Check sheet for the modelled part. Datum: model origin and axes. Units: mm. A direction names the side the tool comes from. Give positions to 0.01 mm unless a question says otherwise; leave off trailing zeros. Order: outer loops, then holes, each group sorted by start corner. A loop starts at its lowest first (then second) coordinate and runs counter-clockwise, first axis right, second up.
```python
from build123d import *

# Parameters (mm, degrees)
F0_R     = 1.5
F1_DEPTH = 2.5
F2_R     = 1


with BuildPart() as f1:
    # F0 (on Front) → F1 (new body)
    with BuildSketch(Plane.XZ):
        with BuildLine():
            ThreePointArc((5, 36.559677), (-0.000826, -36.9), (-4.998364, 36.559901))
            Line((-4.998364, 36.559901), (-5, 36.9))
            Line((-5, 36.9), (-5, 42.204858))
            Line((-5, 42.204858), (-5, 46.9))
            Line((-5, 46.9), (-7.5, 46.9))
            Line((-7.5, 46.9), (-10, 46.9))
            Line((-10, 46.9), (-10, 41.306779))
            ThreePointArc((-10, 41.306779), (0, -42.5), (10, 41.306779))
            Line((10, 41.306779), (10, 46.9))
            Line((10, 46.9), (7.5, 46.9))
            Line((7.5, 46.9), (5, 46.9))
            Line((5, 46.9), (5, 42.204858))
            Line((5, 42.204858), (5, 36.9))
            Line((5, 36.9), (5, 36.559677))
        make_face()
        with Locations((-7.5, 44.552429)):
            Circle(F0_R, mode=Mode.SUBTRACT)
        with Locations((7.5, 44.552429)):
            Circle(F0_R, mode=Mode.SUBTRACT)
    extrude(amount=F1_DEPTH)

    # F2
    f2_edges = [f1.edges().sort_by_distance(p)[0] for p in [
        (-10, -1.25, 46.9),
        (-5, -1.25, 46.9),
        (5, -1.25, 46.9),
        (10, -1.25, 46.9),
        (5, -1.25, 36.559677),
        (-4.998364, -1.25, 36.559901),
    ]]
    fillet(f2_edges, radius=F2_R)


solid = f1.part
```
Q1. Sectioned sample at A-A, the plane z = 0. Record the cut outline in (x, y).
Q2. Sectioned sample at C-C, the plane x = 22. Record the cut outline in (y, z).
Q3. Material ranges on line 1 (Z direction, x = -7.5, y = -0.9); line 2 (X direction, y = -2, z = 0); line 3 (Z direction, x = -28, y = -0.45), recorded low to high.
Q4. Tool access check on faces 4 (the flat face through (-5, -1, 42)), 5 (the flat face through (-10, -1, 44)), 6 (the flat face through (8, -1, 46.9)). Record the directions out of +Z, -Z, +X, -X, +Y, -Y that give a thin tool (end or side, any length) a straight path to the whole face; none if there is none.
Q5. Go/stop test with flat-tipped pins: P1, Ø1.2, axis at y = -1, z = 43, coming from the -X side; P2, Ø0.8, axis at y = -0.5, z = 44, coming from the +X side; P3, Ø0.8, axis at y = -1.5, z = 39.5, coming from the -X side. Record where each tip stops, or that it passes through.
Q6. Sectioned sample at B-B, the plane x = 7.5. Record the cut outline in (y, z).
Q7. Sectioned sample at D-D, the plane y = -1.95. Count the separate pieces of the cut face and the enclosed holes in it, plus the area to 3 significant figures.
Q8. Draft check along X on faces 1 (the flat face through (10, -1, 44)), 2 (the cylindrical face through (-1.727, -1.232, -42.465)), 3 (the flat face through (5, -1, 42)). Enter one of: pulls with the +X half, pulls with the -X half, needs draft (parallel to the pull), parting line crosses it, or undercut.
Filled in:
1. outline: (-42.5, -2.5) - (-36.9, -2.5) - (-36.9, 0) - (-42.5, 0) - close; (36.9, -2.5) - (42.5, -2.5) - (42.5, 0) - (36.9, 0) - close
2. outline: (-2.5, -36.36) - (0, -36.36) - (0, -29.62) - (-2.5, -29.62) - close; (-2.5, 29.62) - (0, 29.62) - (0, 36.36) - (-2.5, 36.36) - close
3. line 1: z = -41.83 to -36.13, 36.13 to 43.05, 46.05 to 46.9
3. line 2: x = -42.5 to -36.9, 36.9 to 42.5
3. line 3: z = -31.97 to -24.03, 24.03 to 31.97
4. face 4: +Z, +Y, -Y
4. face 5: +Z, -X, +Y, -Y
4. face 6: +Z, +X, -X, +Y, -Y
5. P1: stops at x = -10
5. P2: stops at x = 10
5. P3: stops at x = -16.66
6. outline: (-2.5, -41.83) - (0, -41.83) - (0, -36.13) - (-2.5, -36.13) - close; (-2.5, 36.13) - (0, 36.13) - (0, 43.05) - (-2.5, 43.05) - close; (-2.5, 46.05) - (0, 46.05) - (0, 46.9) - (-2.5, 46.9) - close
7. separate pieces: 1
7. enclosed holes: 2
7. area: 1,380 mm2
8. face 1: pulls with the +X half
8. face 2: parting line crosses it
8. face 3: undercut
